from build123d import *

# Parameters (mm, degrees)
F5_DEPTH = 25.4


# Not quite as in the source:
# - the arcs of a loft's sections are written as splines that run evenly, so that the points pair up as in the source's solid


with BuildPart() as f3:
    # F2 (on offset) → F3 section 0
    with BuildSketch(Plane.XY.offset(30.988)):
        Polygon((50.5604938488, 4.6280257192), (27.9056160827, 42.4153126988), (-15.7627597645, 48.2630041015), (-47.5614560073, 17.7676690299), (-43.5454057997, -26.1070832156), (-6.7387768606, -50.3226693123), (35.1422885006, -36.6442590214), align=None)
    # F0 (on Top) → F3 section 1
    with BuildSketch(Plane.XY):
        with BuildLine():
            add(Edge.make_bspline(
                [(29.4866381099, 2.699042457), (29.2174542384, 5.6398362877), (28.5051117676, 8.5396714595), (26.2570337959, 14.0012700055), (24.7215972806, 16.5623070077), (20.9635606735, 21.1186294397), (18.7414603862, 23.1133088958), (16.2744217872, 24.7364074332)],
                knots=[0, 0, 0, 0, 0.3333333333, 0.3333333333, 0.6666666667, 0.6666666667, 1, 1, 1, 1], degree=3))
            add(Edge.make_bspline(
                [(16.2744217872, 24.7364074332), (13.8073831882, 26.3595059706), (11.096062491, 27.6105918574), (5.424359114, 29.2582247193), (2.4647307492, 29.6545525654), (-3.440643072, 29.557221804), (-6.385603136, 29.0635761411), (-9.192766079, 28.1467530815)],
                knots=[0, 0, 0, 0, 0.3333333333, 0.3333333333, 0.6666666667, 0.6666666667, 1, 1, 1, 1], degree=3))
            add(Edge.make_bspline(
                [(-9.192766079, 28.1467530815), (-11.9999290219, 27.2299300218), (-14.6685481598, 25.8901734333), (-19.4929686175, 22.4831394605), (-21.6481283077, 20.4163151987), (-25.2539724079, 15.7386232925), (-26.7041772543, 13.1283777633), (-27.7376135895, 10.3620195702)],
                knots=[0, 0, 0, 0, 0.3333333333, 0.3333333333, 0.6666666667, 0.6666666667, 1, 1, 1, 1], degree=3))
            add(Edge.make_bspline(
                [(-27.7376135895, 10.3620195702), (-28.7710499246, 7.5956613772), (-29.3874428624, 4.6739263506), (-29.7316933959, -1.2222083845), (-29.4595052076, -4.1958239296), (-28.0505454335, -9.9314795677), (-26.9139612341, -12.6927568405), (-25.3954723229, -15.2255260241)],
                knots=[0, 0, 0, 0, 0.3333333333, 0.3333333333, 0.6666666667, 0.6666666667, 1, 1, 1, 1], degree=3))
            add(Edge.make_bspline(
                [(-25.3954723229, -15.2255260241), (-23.8769834116, -17.7582952077), (-21.976993695, -20.0618826048), (-17.5818466312, -24.0072083875), (-15.0872738217, -25.6484220597), (-9.7244856209, -28.1229757482), (-6.8569834599, -28.9559866583), (-3.9300224239, -29.3479399781)],
                knots=[0, 0, 0, 0, 0.3333333333, 0.3333333333, 0.6666666667, 0.6666666667, 1, 1, 1, 1], degree=3))
            add(Edge.make_bspline(
                [(-3.9300224239, -29.3479399781), (-1.003061388, -29.739893298), (1.9825799737, -29.690684771), (7.8074892511, -28.7142908169), (10.6459824762, -27.7872352464), (15.9243102077, -25.1372975861), (18.3634427166, -23.4147679279), (20.4948145181, -21.3707565397)],
                knots=[0, 0, 0, 0, 0.3333333333, 0.3333333333, 0.6666666667, 0.6666666667, 1, 1, 1, 1], degree=3))
            add(Edge.make_bspline(
                [(20.4948145181, -21.3707565397), (22.6261863196, -19.3267451516), (24.449230485, -16.961795725), (27.3176264836, -11.7989265964), (28.3625968311, -9.0016935363), (29.5817756531, -3.2227216343), (29.7558219815, -0.2417513736), (29.4866381099, 2.699042457)],
                knots=[0, 0, 0, 0, 0.3333333333, 0.3333333333, 0.6666666667, 0.6666666667, 1, 1, 1, 1], degree=3))
        make_face()
    loft(ruled=True)

    # F4 (on face) → F5 (cut)
    with BuildSketch(Plane.XY.offset(30.988)):
        Polygon((26.9755858675, 5.5309937743), (15.1636164888, 22.9856228979), (-5.5309937743, 26.9755858675), (-22.9856228979, 15.1636164888), (-26.9755858675, -5.5309937743), (-15.1636164888, -22.9856228979), (5.5309937743, -26.9755858675), (22.9856228979, -15.1636164888), align=None)
    extrude(amount=-F5_DEPTH, mode=Mode.SUBTRACT)


solid = f3.part
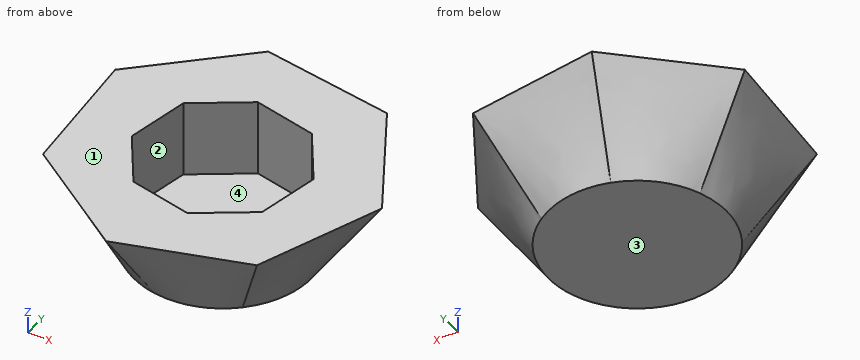
Can you work these out from the model? Positions are in its coordinate system, mm. Face numbers are marked on the shaded views. A direction names the side the tool comes from. Coordinates: 2 decimals unless noted, no trailing zeros. Put each result on its own line as item: value. Start each with the question number.
Item 1: If I drill on line 1 along Y through (x, z) = (9.5, 10); line 2 along Z through (x, y) = (-10.5, 15.5); line 3 along X through (y, z) = (19, 11), over which ranges is the centre line in solid material (lowest first)?
Item 2: Which directions (+Z, -Z, +X, -X, +Y, -Y) give clear straight access to the entire face, cutting with the end or side of a thin tool? Please do the marked faces 3 and 4.
Item 3: For pin 1 (5 mm diameter, centred on y = 7.5, z = 18.5, fed in from +X); pin 2 (2 mm diameter, centred on x = -33.5, z = 20.5, fed in from +Y); pin 3 (3 mm diameter, centred on x = 31, y = -23.5, fed in from -Z), each with a flat end and sliding along its axis, tell me the tip position at first contact or that it passes through.
Item 4: If we mould it in two halves opening along X, with no side actions, what happens to the marked faces 1 and 2? For each: +X half, -X half, draft (parallel to the pull), parting line (faces both ways), or undercut.
Here are the results:
1. line 1: -33.51 to -24.29, 24.08 to 33.66
1. line 2: 0 to 5.59
1. line 3: -30.43 to -17.32, 17.86 to 29.8
2. face 3: -Z, +X, -X, +Y, -Y
2. face 4: +Z
3. pin 1: x = 42.47
3. pin 2: y = 24.74
3. pin 3: z = 13.22
4. face 1: draft
4. face 2: undercut
